Here's how the part is built. I have some questions about the finished solid (model axes, mm). Face numbers are marked on the shaded views. Give positions to 0.01 mm unless a question says otherwise; leave off trailing zeros. Write each loop counter-clockwise with the first axis right and the second up, starting at its lowest first coordinate (ties: lowest second). Pieces come first, ordered by that corner, then holes. Notation, with made-up numbers: M -17.75,30 L 23.25,30 A25 ccw 23.25,58 Z; hole C -11.75,10 d10. An arc over 180 degrees is marked long. Answer as CSV lines item,"result". Start each with the question number.
Q1. Suppose I cut it at A-A (x = 3). Write out the boundary of the cut face in (y, z).
Q2. Thinking about a two-plate mould opening in Z: for the marked faces 1, 2 and 3, which applies, +Z half, -Z half, draft (parallel to the pull), parting line (faces both ways), or undercut?
Q3. If I drill on line 1 along Z through (x, y) = (3, 3.5); line 2 along Z through (x, y) = (3, -7.5); line 3 along X through (y, z) = (-11, -16), over which ranges is the centre line in solid material (lowest first)?
Q4. For pin 1 (5 mm diameter, centred on y = 11.5, z = -6, fed in from +X); pin 2 (2 mm diameter, centred on x = 2, z = 12.5, fed in from +Y); pin 3 (2 mm diameter, centred on x = 5, y = -6, fed in from -Z); pin 4 (2 mm diameter, centred on x = 1.5, y = -0.5, fed in from -Z), each with a flat end and sliding along its axis, tell me the tip position at first contact or that it passes through.
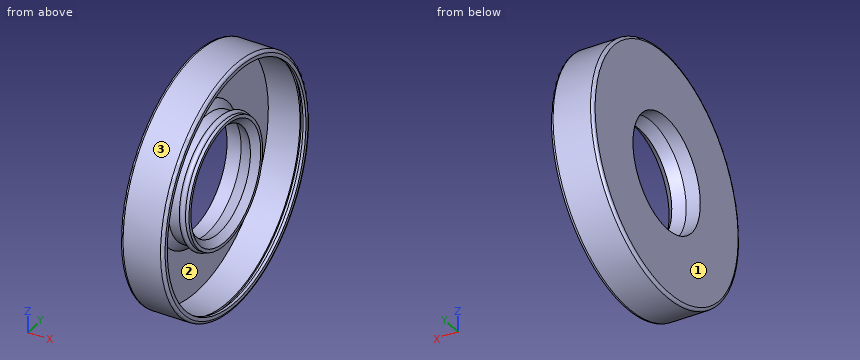
```python
from build123d import *


with BuildPart() as part:
    # Esquisse1 → Base-Révolution (revolve)
    with BuildSketch(Plane(origin=(0, 0, 0), x_dir=(1, 0, 0), z_dir=(0, 1, 0)), mode=Mode.PRIVATE) as base_r_volution_sk:
        with BuildLine():
            Line((0, 9.2), (0, 19.533333333))
            ThreePointArc((0, 19.533333333), (0.136683502, 19.863316498), (0.466666667, 20))
            Line((0.466666667, 20), (6.533333333, 20))
            ThreePointArc((6.533333333, 20), (6.863316498, 19.863316498), (7, 19.533333333))
            Line((7, 19.533333333), (7, 18.95))
            Line((7, 18.95), (6.533333333, 18.95))
            Line((6.533333333, 18.95), (6.533333333, 19.65))
            Line((6.533333333, 19.65), (5.833333333, 19.65))
            Line((5.833333333, 19.65), (5.833333333, 19.3))
            Line((5.833333333, 19.3), (0.7, 19.3))
            Line((0.7, 19.3), (0.7, 11.151341272))
            Line((0.7, 11.151341272), (1.75, 9.9))
            Line((1.75, 9.9), (3.675, 9.9))
            ThreePointArc((3.675, 9.9), (4.111221461, 10.417439244), (4.694974747, 10.075))
            Line((4.694974747, 10.075), (5.25, 10.075))
            Line((5.25, 10.075), (5.25, 9.55))
            Line((5.25, 9.55), (4.2, 8.5))
            Line((4.2, 8.5), (2.276765806, 9.2))
            Line((2.276765806, 9.2), (0, 9.2))
        make_face()
    revolve(base_r_volution_sk.sketch.rotate(Axis((0, 0, 0), (1, 0, 0)), 180), axis=Axis((0, 0, 0), (1, 0, 0)))


solid = part.part
```
Resolved:
1,outline,"C 0,0 d40; C 0,0 d19.8; hole C 0,0 d38.6; hole C 0,0 d17.87"
2,face 1,"draft"
2,face 2,"undercut"
2,face 3,"parting line"
3,line 1,"-19.69 to -18.98, -9.26 to -8.22, 8.22 to 9.26, 18.98 to 19.69"
3,line 2,"-18.54 to -17.78, -6.46 to -4.86, 4.86 to 6.46, 17.78 to 18.54"
3,line 3,"0 to 5.83, 6.53 to 7"
4,pin 1,"x = 1.27"
4,pin 2,"y = 16.36"
4,pin 3,"z = -19.36"
4,pin 4,"z = -20"
